```python
from build123d import *

# Parameters (mm, degrees)
BOSS_EXTRUDE1_DEPTH      = 381
SKETCH3_W                = 98.988046958
SKETCH3_H                = 406.4
SKETCH3_H_2              = 101.6
CUT_EXTRUDE1_DEPTH       = 121.65
CUT_EXTRUDE1_DEPTH_BACK  = 57.038415052
BOSS_EXTRUDE2_DEPTH      = 152.4
CUT_EXTRUDE2_DEPTH       = 252.388046958
CUT_EXTRUDE2_DEPTH_BACK  = 1
CUT_EXTRUDE3_DEPTH       = 121.65
CUT_EXTRUDE3_DEPTH_BACK  = 57.038415052
SKETCH8_W                = 63.5
SKETCH8_H                = 19.05
BOSS_EXTRUDE3_DEPTH      = 730.25
BOSS_EXTRUDE3_DEPTH_BACK = 431.8
FILLET1_R                = 25.4
BOSS_EXTRUDE4_DEPTH      = 704.85
BOSS_EXTRUDE4_DEPTH_BACK = 406.4
SKETCH10_R               = 25.4
BOSS_EXTRUDE5_DEPTH      = 50.8


with BuildPart() as part:
    # Sketch2 → Boss-Extrude1 (new body, symmetric)
    with BuildSketch(Plane.XY):
        Polygon((152.4, 0), (0, 0), (0, 120.65), (101.6, 120.65), (152.4, 82.55), (152.4, 69.85), (251.388046958, 20.161584948), (251.388046958, -56.038415052), (228.6, -56.038415052), (228.6, -12.7), (165.1, -12.7), (165.1, -50.8), (152.4, -50.8), align=None)
    extrude(amount=BOSS_EXTRUDE1_DEPTH, both=True)

    # Sketch3 → Cut-Extrude1 (cut, two sides)
    with BuildSketch(Plane(origin=(0, 0, 0), x_dir=(1, 0, 0), z_dir=(0, 1, 0))) as cut_extrude1_sk:
        with Locations((201.894023479, -76.2)):
            Rectangle(SKETCH3_W, SKETCH3_H)
        with Locations((201.894023479, 279.4)):
            Rectangle(SKETCH3_W, SKETCH3_H_2)
    extrude(amount=CUT_EXTRUDE1_DEPTH, mode=Mode.SUBTRACT)
    extrude(cut_extrude1_sk.sketch, amount=-CUT_EXTRUDE1_DEPTH_BACK, mode=Mode.SUBTRACT)

    # Sketch4 → Boss-Extrude2 (add)
    with BuildSketch(Plane.XY.offset(381)):
        Polygon((152.4, 0), (0, 0), (0, 101.6), (95.25, 101.6), (152.4, 58.7375), align=None)
    extrude(amount=BOSS_EXTRUDE2_DEPTH)

    # Sketch6 → Cut-Extrude2 (cut, two sides)
    with BuildSketch(Plane(origin=(0, 0, 0), x_dir=(0, 0, -1), z_dir=(1, 0, 0))) as cut_extrude2_sk:
        Polygon((-533.4, 101.6), (-533.4, 58.7375), (-457.2, 101.6), align=None)
    extrude(amount=CUT_EXTRUDE2_DEPTH, mode=Mode.SUBTRACT)
    extrude(cut_extrude2_sk.sketch, amount=-CUT_EXTRUDE2_DEPTH_BACK, mode=Mode.SUBTRACT)

    # Sketch7 → Cut-Extrude3 (cut, two sides)
    with BuildSketch(Plane(origin=(0, 0, 0), x_dir=(1, 0, 0), z_dir=(0, 1, 0))) as cut_extrude3_sk:
        Polygon((152.4, -533.4), (152.4, -457.2), (95.25, -533.4), align=None)
    extrude(amount=CUT_EXTRUDE3_DEPTH, mode=Mode.SUBTRACT)
    extrude(cut_extrude3_sk.sketch, amount=-CUT_EXTRUDE3_DEPTH_BACK, mode=Mode.SUBTRACT)

    # Mirror1: part across plane


with BuildPart() as part_1:
    add(part.part)
    add(part.part.mirror(Plane(origin=(0, 0, 0), x_dir=(0, 0, 1), z_dir=(1, 0, 0))))

    # Sketch8 → Boss-Extrude3 (add, two sides)
    with BuildSketch(Plane.XY) as boss_extrude3_sk:
        with Locations((-196.85, -22.225)):
            Rectangle(SKETCH8_W, SKETCH8_H)
        with Locations((196.85, -22.225)):
            Rectangle(SKETCH8_W, SKETCH8_H)
    extrude(amount=BOSS_EXTRUDE3_DEPTH)
    extrude(boss_extrude3_sk.sketch, amount=-BOSS_EXTRUDE3_DEPTH_BACK)

    # Fillet1
    fillet1_edges = [part_1.edges().sort_by_distance(p)[0] for p in [
        (-165.1, -22.225, 730.25),
        (-228.6, -22.225, 730.25),
        (-228.6, -22.225, -431.8),
        (-165.1, -22.225, -431.8),
        (228.6, -22.225, 730.25),
        (165.1, -22.225, 730.25),
        (165.1, -22.225, -431.8),
        (228.6, -22.225, -431.8),
    ]]
    fillet(fillet1_edges, radius=FILLET1_R)

    # Sketch9 → Boss-Extrude4 (add, two sides)
    with BuildSketch(Plane.XY) as boss_extrude4_sk:
        Polygon((177.8, -50.8), (215.9, -50.8), (215.9, -44.45), (209.55, -44.45), (209.55, -31.75), (184.15, -31.75), (184.15, -44.45), (177.8, -44.45), align=None)
        Polygon((-184.15, -44.45), (-184.15, -31.75), (-209.55, -31.75), (-209.55, -44.45), (-215.9, -44.45), (-215.9, -50.8), (-177.8, -50.8), (-177.8, -44.45), align=None)
    extrude(amount=BOSS_EXTRUDE4_DEPTH)
    extrude(boss_extrude4_sk.sketch, amount=-BOSS_EXTRUDE4_DEPTH_BACK)

    # Sketch10 → Boss-Extrude5 (add)
    with BuildSketch(Plane(origin=(0, 120.65, 0), x_dir=(1, 0, 0), z_dir=(0, 1, 0))):
        with Locations((0, 177.8)):
            Circle(SKETCH10_R)
        with Locations((0, -127)):
            Circle(SKETCH10_R)
    extrude(amount=BOSS_EXTRUDE5_DEPTH)


solid = part_1.part
```
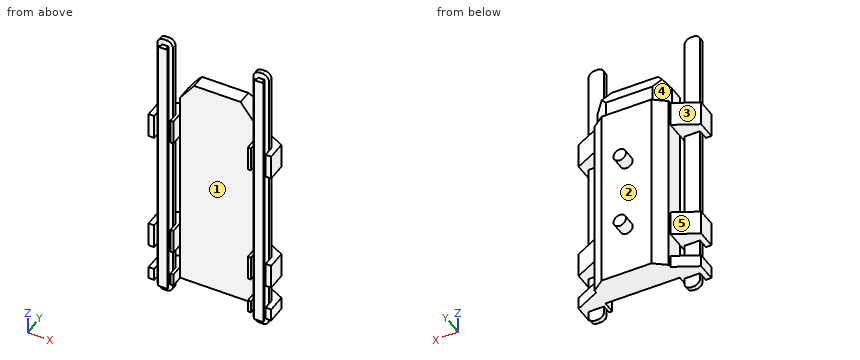
Here's how the part is built. I have some questions about the finished solid (model axes, mm). Face numbers are marked on the shaded views. A direction names the side the tool comes from. Round coordinates to 2 decimals unless told otherwise and drop trailing zeros. Order: outer loops, then holes, each group sorted by start corner. A loop starts at its lowest first (then second) coordinate and runs counter-clockwise, first axis right, second up. Notation, with made-up numbers: M -34,-35.5 L -26,-35.5 A19 cw -26,-29.5 Z; hole C -8,-3.5 d8. An arc over 180 degrees is marked long. Answer in a Markdown table with one row per item.
Item 1: For the marked faces 4 and 5, which set-ups out of +Z, -Z, +X, -X, +Y, -Y let a thin tool reach every point of the face, with its end or its side?
A:
| item | result |
|---|---|
| face 4 | +Z, -X, +Y |
| face 5 | +Z, -Z, -X, +Y |
Item 2: Imagine slicing it at C-C, the plane y = 143. Write out the boundary of the cut face in (x, z).
A:
| item | result |
|---|---|
| outline | C 0,-177.8 d50.8; C 0,127 d50.8 |
Item 3: I'm going to push flat-ended pins straight in: pin 1 (4 mm diameter, centred on x = 31.5, y = 58, fed in from -Z); pin 2 (2 mm diameter, centred on x = 52, y = 75, fed in from +Z); pin 3 (4 mm diameter, centred on x = 180, y = -19.5, fed in from +Z). Where does each tip first touch, or does it pass through?
A:
| item | result |
|---|---|
| pin 1 | stops at z = -381 |
| pin 2 | stops at z = 506.27 |
| pin 3 | stops at z = 728.79 |
Item 4: Imagine slicing it at B-B, the plane x = -55.5. Write out the boundary of the cut face in (y, z).
A:
| item | result |
|---|---|
| outline | M 0,-381 L 120.65,-381 L 120.65,381 L 101.6,381 L 101.6,457.2 L 58.74,533.4 L 0,533.4 Z |
Item 5: If I drill on L1, parallel to Z at x = 186, y = -4.5; L2, parallel to X at y = -38.5, z = 399; L3, parallel to Y at x = -175, z = 227.5, over which ranges is the centre line in solid material (lowest first)? Write a range as from..to.
A:
| item | result |
|---|---|
| L1 | z = -381..-330.2, -228.6..-127, 279.4..381 |
| L2 | x = -209.55..-184.15, 184.15..209.55 |
| L3 | y = -31.75..-12.7 |
Item 6: Thinking about a two-plate mould opening in X: for the marked faces 1, 2 and 3, which applies, +X half, -X half, draft (parallel to the pull), parting line (faces both ways), or undercut?
A:
| item | result |
|---|---|
| face 1 | undercut |
| face 2 | draft |
| face 3 | -X half |
Item 7: Imagine slicing it at A-A, the plane z = 127. State how many separate pieces and enclosed holes the cut face has, and give its area (3 significant figures).
A:
| item | result |
|---|---|
| separate pieces | 3 |
| enclosed holes | 0 |
| area | 41,000 mm2 |
